```python
from build123d import *

# Parameters (mm, degrees)
SKETCH1_W           = 59
SKETCH1_H           = 21
SKETCH1_R           = 1.75
BOSS_EXTRUDE1_DEPTH = 7
SKETCH2_W           = 59
SKETCH2_H           = 5
BOSS_EXTRUDE2_DEPTH = 155
CUT_EXTRUDE1_DEPTH  = 159.591456264
FILLET1_R           = 3
FILLET2_R           = 3


with BuildPart() as part:
    # Sketch1 → Boss-Extrude1 (new body)
    with BuildSketch(Plane.XY):
        with Locations((0, -2.5)):
            Rectangle(SKETCH1_W, SKETCH1_H)
        with Locations((-17, 0)):
            Circle(SKETCH1_R, mode=Mode.SUBTRACT)
        with Locations((17, 0)):
            Circle(SKETCH1_R, mode=Mode.SUBTRACT)
    extrude(amount=BOSS_EXTRUDE1_DEPTH)

    # Sketch2 → Boss-Extrude2 (add)
    with BuildSketch(Plane(origin=(0, 0, 0), x_dir=(-1, 0, 0), z_dir=(0, 0, -1))):
        with Locations((0, -10.5)):
            Rectangle(SKETCH2_W, SKETCH2_H)
    extrude(amount=BOSS_EXTRUDE2_DEPTH)

    # Sketch4 → Cut-Extrude1 (cut, through all)
    with BuildSketch(Plane(origin=(0, -8, 0), x_dir=(1, 0, 0), z_dir=(0, 1, 0))):
        with BuildLine():
            Line((-15.5, 155), (15.5, 155))
            ThreePointArc((15.5, 155), (0, 139.5), (-15.5, 155))
        make_face()
    extrude(amount=-CUT_EXTRUDE1_DEPTH, mode=Mode.SUBTRACT)

    # Fillet1
    fillet1_edges = [part.edges().sort_by_distance(p)[0] for p in [
        (0, -8, 0),
    ]]
    fillet(fillet1_edges, radius=FILLET1_R)

    # Fillet2
    fillet2_edges = [part.edges().sort_by_distance(p)[0] for p in [
        (29.5, -10.5, -155),
        (-29.5, -10.5, -155),
        (15.5, -10.5, -155),
        (-15.5, -10.5, -155),
    ]]
    fillet(fillet2_edges, radius=FILLET2_R)


solid = part.part
```
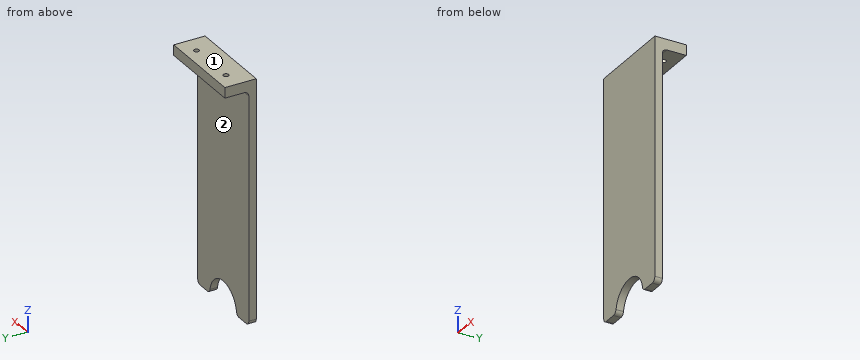
Can you work these out from the model? Positions are in its coordinate system, mm. Face numbers are marked on the shaded views. A direction names the side the tool comes from. Round coordinates to 2 decimals unless told otherwise and drop trailing zeros. Loops run counter-clockwise (first coordinate to the right, second up) from the corner with the lowest first, then second, coordinate; pieces in that order, holes last. Notation, with made-up numbers: M 62,56 L 102,56 A28 ccw 102,94 Z; hole C 9.25,60.5 d9. An arc over 180 degrees is marked long. Write item = value, one per line. Start each with the question number.
(1) I'm going to push flat-ended pins straight in: P1, Ø5, axis at x = -18.5, z = -125, coming from the +Y side; P2, Ø6.5, axis at x = 13.5, y = 4, coming from the -Z side. Where does each tip first touch, or does it pass through?
(2) Suppose I cut it at A-A on y = 0. Write out the boundary of the cut face in (x, z).
(3) Suppose I cut it at D-D on y = -9.5. Write out the boundary of the cut face in (x, z).
(4) Suppose I cut it at B-B on x = -23. Write out the boundary of the cut face in (y, z).
(5) Which directions (+Z, -Z, +X, -X, +Y, -Y) give clear straight access to the entire face, cutting with the end or side of a thin tool? Please do the marked faces 1 and 2.
(6) I need wall thicknesses on line 1 along Y through (x, z) = (-17, 4); line 2 along Y through (x, z) = (-1, -54.5); line 3 along Z through (x, y) = (11, -0.5). Which ranges of each line are inside material? Lowest first, please.
(7) Suppose I cut it at C-C on z = -145. Write out the boundary of the cut face in (x, y), plus the area to 3 significant figures.
Answer block:
q1.P1 = -8
q1.P2 = 0
q2.outline = M -29.5,0 L -18.75,0 L -18.75,7 L -29.5,7 Z; M -15.25,0 L 15.25,0 L 15.25,7 L -15.25,7 Z; M 18.75,0 L 29.5,0 L 29.5,7 L 18.75,7 Z
q3.outline = M -29.5,-152 A3 ccw -26.5,-155 L -18.26,-155 A3 ccw -15.29,-152.49 A15.5 cw 15.29,-152.49 A3 ccw 18.26,-155 L 26.5,-155 A3 ccw 29.5,-152 L 29.5,7 L -29.5,7 Z
q4.outline = M -13,-155 L -8,-155 L -8,-3 A3 cw -5,0 L 8,0 L 8,7 L -13,7 Z
q5.face_1 = +Z, +X, -X, +Y, -Y
q5.face_2 = -Z, +X, -X, +Y
q6.line_1 = -13 to -1.75, 1.75 to 8
q6.line_2 = -13 to -8
q6.line_3 = 0 to 7
q7.outline = M -29.5,-13 L -11.84,-13 L -11.84,-8 L -29.5,-8 Z; M 11.84,-13 L 29.5,-13 L 29.5,-8 L 11.84,-8 Z
q7.area = 177 mm²
